Autodesk Inventor part; units mm, degrees
ref_plane "YZ Plane" through (0, 0, 0) normal (1, 0, 0) x (0, 1, 0)
ref_plane "XZ Plane" through (0, 0, 0) normal (0, 1, 0) x (-1, 0, 0)
ref_plane "XY Plane" through (0, 0, 0) normal (0, 0, 1) x (1, 0, 0)
sketch "Skizze1" plane through (0, 0, 0) normal (0, 1, 0) x (-1, 0, 0)
  line L0 (-27, 27) -> (27, 27)
  line L1 (27, 27) -> (27, -27)
  line L2 (27, -27) -> (-27, -27)
  line L3 (-27, -27) -> (-27, 27)
  line L4 (-27, 27) -> (27, -27) construction
  line L5 (27, 27) -> (-27, -27) construction
  point P0 (0, 0)
  dimension "d0" = 54
  dimension "d1" = 54
extrude "Extrusion1" add sketch "Skizze1" along normal blind 95
sketch "Skizze2" plane through (27, 0, 27) normal (1, 0, 0) x (0, 0, -1)
  line L0 (5, 0) -> (49, 0)
  line L1 (49, 0) -> (49, 95)
  line L2 (49, 95) -> (5, 95)
  line L3 (5, 95) -> (5, 0)
  line L4 (0, 0) -> (0, 95)
  line L5 (54, 0) -> (54, 95)
  line L6 (54, 0) -> (0, 0)
  line L7 (54, 0) -> (54, 95)
  line L8 (0, 95) -> (54, 95)
  line L9 (0, 0) -> (0, 95)
  line L10 (0, 95) -> (54, 95)
  line L11 (54, 0) -> (0, 0)
  point P0 (27, 0)
  dimension "d4" = 5
  dimension "d5" = 5
extrude "Extrusion2" cut sketch "Skizze2" against normal blind 49 contours L3 L2 L1 L0
sketch "Skizze3" plane through (27, 0, -27) normal (0, 0, -1) x (-1, 0, 0)
  line L0 (54, 0) -> (0, 0)
  line L1 (54, 0) -> (54, 95)
  line L2 (0, 95) -> (54, 95)
  line L3 (0, 0) -> (0, 95)
  line L4 (61.4003, 122.4392) -> (0, 47.227)
  line L5 (0, 47.227) -> (39, 95)
  line L6 (39, 95) -> (33.5775, 99.4267) construction
  line L7 (33.5775, 99.4267) -> (-5.4225, 51.6538) construction
  line L8 (-5.4225, 51.6538) -> (0, 47.227) construction
  line L9 (31.8094, 54.61) -> (-25.1559, 101.1143) construction
  line L10 (27.9901, 92.5825) -> (-13.8409, 126.7317)
  line L11 (-13.8409, 126.7317) -> (-47.9901, 84.9007)
  line L12 (-47.9901, 84.9007) -> (-6.1591, 50.7515) construction
  line L13 (-6.1591, 50.7515) -> (27.9901, 92.5825) construction
  line L14 (27.9901, 92.5825) -> (-47.9901, 84.9007) construction
  line L15 (-13.8409, 126.7317) -> (-6.1591, 50.7515) construction
  line L16 (0, 95) -> (54, 95)
  point P0 (27, 0)
  point P1 (-10, 88.7416)
  point P2 (-10, 88.7416)
  dimension "d34" = 7
  dimension "d35" = 61.6706
  dimension "d36" = 25.8353
  dimension "d37" = 54
  dimension "d38" = 54
  dimension "d39" = 15
  dimension "d60" = 10
extrude "Extrusion3" cut sketch "Skizze3" against normal through all contours L3 L2 L4
sketch "Skizze4" plane through (27, 0, -27) normal (0, 0, -1) x (-1, 0, 0)
  line L0 (9.5, 6.25) -> (44.5, 6.25)
  line L1 (44.5, 6.25) -> (44.5, 33.75)
  line L2 (44.5, 33.75) -> (9.5, 33.75)
  line L3 (9.5, 33.75) -> (9.5, 6.25)
  line L4 (9.5, 6.25) -> (44.5, 33.75) construction
  line L5 (44.5, 6.25) -> (9.5, 33.75) construction
  line L6 (27, 0) -> (27, 60.1271) construction
  line L7 (54, 0) -> (0, 0) construction
  point P0 (27, 20)
  point P1 (27, 20)
  dimension "d11" = 35
  dimension "d12" = 27.5
  dimension "d62" = 20
hole "Bohrung1" at (17.5, 33.75, -27) at (-17.5, 33.75, -27) at (-17.5, 6.25, -27) at (0, 20, -27) at (17.5, 6.25, -27) direction (0, 0, 1) diameter 2.459 end up to surface
sketch "Skizze5" plane through (27, 47.227, -22) normal (0.7746482, 0.6323925, 0) x (0, 0, -1)
  line L0 (-49, 0) -> (-49, 61.6706)
  line L1 (-44, 0) -> (-49, 0)
  line L2 (-44, 61.6706) -> (-44, 0)
  line L3 (0, 61.6706) -> (5, 61.6706)
  line L4 (0, 0) -> (0, 61.6706)
  line L5 (5, 0) -> (0, 0)
  line L6 (5, 61.6706) -> (5, 0)
  line L7 (0, 61.6706) -> (5, 61.6706)
  line L8 (-49, 0) -> (-49, 61.6706)
  line L9 (-44, 0) -> (-49, 0)
  line L10 (-44, 61.6706) -> (-44, 0)
  line L11 (-49, 61.6706) -> (-44, 61.6706)
  line L12 (0, 0) -> (0, 61.6706)
  line L13 (5, 0) -> (0, 0)
  line L14 (5, 61.6706) -> (5, 0)
  line L15 (-49, 61.6706) -> (-44, 61.6706)
  point P0 (127.5861, 27)
  point P1 (-46.5, 55)
  point P2 (2.5, 55)
  dimension "d41" = 2.5
  dimension "d42" = 2.5
  dimension "d43" = 55
  dimension "d44" = 55
hole "Bohrung2" [suppressed]
pattern_linear "Rechteckige Anordnung1" [suppressed]
pattern_circular "Runde Anordnung1" count 3 over 180 about axis through (0, -10, 0) along (0, 1, 0) of "Bohrung1"
sketch "Skizze6" plane through (-27, 0, 27) normal (0, 0, 1) x (1, 0, 0)
  circle A0 centre (27, 20) radius 1.2295
  circle A1 centre (9.5, 6.25) radius 1.2295
  circle A2 centre (44.5, 6.25) radius 1.2295
  circle A3 centre (9.5, 33.75) radius 1.2295
  circle A4 centre (44.5, 33.75) radius 1.2295
  line L0 (54, 47.227) -> (15, 95)
  line L1 (0, 95) -> (15, 95)
  line L2 (0, 0) -> (0, 95)
  line L3 (54, 0) -> (0, 0)
  line L4 (54, 0) -> (54, 47.227)
  line L5 (5, 95) -> (5, 0) construction
  line L6 (15, 95) -> (-19.3701, 66.9416) construction
  line L7 (54, 47.227) -> (15, 95) construction
  point P0 (27, 0)
  point P1 (27.4648, 71.8248)
  dimension "d48" = 5
  dimension "d49" = 25.8353
  dimension "d61" = 61.6706
hole "Bohrung3" at (0.4648, 71.8248, 27) direction (0, 0, -1) diameter 2.459 end through all
pattern_linear "Rechteckige Anordnung2" count 3 spacing 20 along (-0.6323925, 0.7746482, 0) of "Bohrung3" first direction both ways yes
properties part number "complex_cube" material "Aluminium 6061"
Verification items for the finished model (mm, model axes). A direction names the side the tool comes from. Coordinates: 2 decimals unless noted, no trailing zeros. Order: outer loops, then holes, each group sorted by start corner. A loop starts at its lowest first (then second) coordinate and runs counter-clockwise, first axis right, second up. Notation, with made-up numbers: (64.25, 8.5) -> (95.25, 8.5) arc R27 cw to (95.25, 44.5) -> close; hole circle Ø6 at (54.25, 10). An arc over 180 degrees is marked (long way). Put each result on its own line as item: value. Start each with the question number.
1) Release check for a two-part mould opening along Z. For faces 1 (the cylindrical face through (-24.465, 32.713, -16.839)), 2 (the flat face through (0, 36, -27)), 3 (the cylindrical face through (-18.331, 5.344, -24.465)) record: pulls with the +Z half, pulls with the -Z half, needs draft (parallel to the pull), parting line crosses it, or undercut.
2) Tool access check on faces 4 (the flat face through (-3, 36, -22)), 5 (the cylindrical face through (16.669, 5.344, -24.465)). Record the directions out of +Z, -Z, +X, -X, +Y, -Y that give a thin tool (end or side, any length) a straight path to the whole face; none if there is none.
3) Cross-section at B-B (y = 20). Enter the section's corners in (x, z), plus the area to 3 significant figures.
4) Go/stop test with a flat-tipped pin: pin 1 (8 mm diameter, centred on y = 83, z = -17, fed in from +X). Record where the tip stops, or that it passes through.
5) Material ranges on L1, parallel to Y at x = -23.25, z = -17.5; L2, parallel to X at y = 33.75, z = 25.65; L3, parallel to Z at x = -25, y = 33, recorded low to high.
6) Cross-section at D-D (z = -17.5). Enter the section's corners in (x, y), plus the area to 3 significant figures.
7) Cross-section at C-C (x = 21). Enter the section's corners in (y, z), plus the area to 3 significant figures.
8) Cross-section at A-A (z = 0). Enter the section's corners in (x, y), plus the area to 3 significant figures.
Geometry check:
1. face 1: undercut
1. face 2: pulls with the -Z half
1. face 3: needs draft
2. face 4: +X, +Y, -Y
2. face 5: +Z, -Z
3. outline: (-27, -27) -> (-1.23, -27) -> (-1.23, -22) -> (-22, -22) -> (-22, -1.23) -> (-27, -1.23) -> close; (-27, 1.23) -> (-22, 1.23) -> (-22, 22) -> (-1.23, 22) -> (-1.23, 27) -> (-27, 27) -> close; (1.23, -27) -> (27, -27) -> (27, -22) -> (1.23, -22) -> close; (1.23, 22) -> (27, 22) -> (27, 27) -> (1.23, 27) -> close
3. area: 723 mm^2
4. pin 1: stops at x = -22
5. L1: y = 0 to 5.02, 7.48 to 32.52, 34.98 to 95
5. L2: x = -27 to -18.73, -16.27 to 16.27, 18.73 to 27
5. L3: z = -27 to -18.47, -16.53 to 16.53, 18.47 to 27
6. outline: (-27, 0) -> (-22, 0) -> (-22, 5.02) -> (-27, 5.02) -> close; (-27, 7.48) -> (-22, 7.48) -> (-22, 32.52) -> (-27, 32.52) -> close; (-27, 34.98) -> (-22, 34.98) -> (-22, 95) -> (-27, 95) -> close
6. area: 450 mm^2
7. outline: (0, -27) -> (54.58, -27) -> (54.58, -22) -> (0, -22) -> close; (0, 22) -> (54.58, 22) -> (54.58, 27) -> (0, 27) -> close
7. area: 546 mm^2
8. outline: (-27, 0) -> (-22, 0) -> (-22, 18.77) -> (-27, 18.77) -> close; (-27, 21.23) -> (-22, 21.23) -> (-22, 95) -> (-27, 95) -> close
8. area: 463 mm^2
